The model under review builds one solid part; all positions refer to its coordinate system, in mm. A direction names the side the tool comes from. Round coordinates to 2 decimals unless told otherwise and drop trailing zeros. Order: outer loops, then holes, each group sorted by start corner. A loop starts at its lowest first (then second) coordinate and runs counter-clockwise, first axis right, second up.
1) Mouldability with a two-part tool opening along Z and no side actions: class faces 1 (the face through (30.04, 1.23, 95.38)), 2 (the face through (36, -4, 57.891)), 3 (the face through (-58.047, 1.268, -52.401)) as pulls with the +Z half, pulls with the -Z half, needs draft (parallel to the pull), parting line crosses it, or undercut.
2) Consider section A-A (z = -79). Give the boundary of the cut face in (x, y).
3) To check wall thickness, follow L1, parallel to X at y = 2, z = -38; L2, parallel to Z at x = 14.51, y = 3.95; L3, parallel to Z at x = -30.5, y = 0.5. State the ranges of each line that lie inside material, in increasing order.
4) Consider section B-B (z = 37). Give the number of separate pieces and of enclosed holes in the cut face, then the cut area to 3 significant figures.
5) Clearance check with flat-ended pins moving along their axes: P1, Ø5, axis at x = 13.5, z = -23.5, coming from the -Y side; P2, Ø1.2, axis at x = 37.5, y = 1, coming from the -Z side; P3, Ø1.5, axis at y = 3, z = 26, coming from the -X side. State where each tip first meets the part, or that it passes through.
6) Machinability: for faces 4 (the face through (39, -3, 43)), 5 (the face through (-36.06, 1.27, 35.72)), 6 (the face through (0, 1, -55)), 7 (the face through (14, 5, 6.35)), which of the approach directions +Z, -Z, +X, -X, +Y, -Y give a long, thin tool a straight path to every point of the face, cutting with its end or side? Answer none if there is none.
from build123d import *

# Parameters (mm, degrees)
IZIM1_R                     = 100
IZIM1_W                     = 64
IZIM1_H                     = 64
Y_KSEKLIK_EKSTR_ZYON1_DEPTH = 2.5
KES_EKSTR_ZYON1_DEPTH       = 142.443451598
IZIM3_W                     = 4.7
IZIM3_H                     = 12.7
IZIM3_R                     = 1
Y_KSEKLIK_EKSTR_ZYON2_DEPTH = 5.85
IZIM4_W                     = 4
IZIM4_H                     = 30
Y_KSEKLIK_EKSTR_ZYON3_DEPTH = 4
Y_KSEKLIK_EKSTR_ZYON4_START = 4
IZIM4_3_W                   = 3
IZIM4_3_H                   = 30
IZIM4_3_W_2                 = 4
Y_KSEKLIK_EKSTR_ZYON4_DEPTH = 3
IZIM5_R                     = 3
Y_KSEKLIK_EKSTR_ZYON5_DEPTH = 3
Y_KSEKLIK_EKSTR_ZYON6_START = 3
IZIM5_3_R                   = 5
Y_KSEKLIK_EKSTR_ZYON6_DEPTH = 2
IZIM11_R                    = 1
KES_EKSTR_ZYON5_DEPTH       = 142.667648036
IZIM12_R                    = 5.7
KES_EKSTR_ZYON6_DEPTH       = 142.667648036
KES_EKSTR_ZYON7_DEPTH       = 142.740079018
KES_EKSTR_ZYON8_DEPTH       = 40


with BuildPart() as part:
    # Çizim1 → Yükseklik-Ekstrüzyon1 (new body)
    with BuildSketch(Plane(origin=(0, 0, 0), x_dir=(1, 0, 0), z_dir=(0, 1, 0))):
        with Locations(Location((0, 0, 0), (0, 0, 270))):
            Circle(IZIM1_R)
        with Locations((0, -48)):
            Rectangle(IZIM1_W, IZIM1_H, mode=Mode.SUBTRACT)
    extrude(amount=Y_KSEKLIK_EKSTR_ZYON1_DEPTH)

    # Çizim2 → Kes-Ekstrüzyon1 (cut, through all)
    with BuildSketch(Plane.XZ):
        with BuildLine():
            ThreePointArc((1.17075, 1.767705982), (-11.89, 0), (1.17075, -1.767705982))
            ThreePointArc((1.17075, -1.767705982), (2.785, 0), (1.17075, 1.767705982))
        make_face()
        with BuildLine():
            ThreePointArc((0.78075, 1.254220649), (-11.39, 0), (0.78075, -1.254220649))
            ThreePointArc((0.78075, -1.254220649), (2.285, 0), (0.78075, 1.254220649))
        make_face(mode=Mode.SUBTRACT)
        with BuildLine():
            ThreePointArc((0.78075, -1.254220649), (2.285, 0), (0.78075, 1.254220649))
            ThreePointArc((0.78075, 1.254220649), (-11.39, 0), (0.78075, -1.254220649))
        make_face()
    extrude(amount=-KES_EKSTR_ZYON1_DEPTH, mode=Mode.SUBTRACT)

    # Çizim3 → Yükseklik-Ekstrüzyon2 (add)
    with BuildSketch(Plane(origin=(0, 2.5, 0), x_dir=(1, 0, 0), z_dir=(0, 1, 0))):
        with Locations((-14.24, 0)):
            Rectangle(IZIM3_W, IZIM3_H)
        with Locations((-14.49, 0)):
            Circle(IZIM3_R, mode=Mode.SUBTRACT)
        with Locations((14.26, 0)):
            Rectangle(IZIM3_W, IZIM3_H)
        with Locations((14.51, 0)):
            Circle(IZIM3_R, mode=Mode.SUBTRACT)
    extrude(amount=Y_KSEKLIK_EKSTR_ZYON2_DEPTH)

    # Çizim4 → Yükseklik-Ekstrüzyon3 (add)
    with BuildSketch(Plane.XZ):
        with Locations((37, 42.891487162)):
            Rectangle(IZIM4_W, IZIM4_H)
    extrude(amount=Y_KSEKLIK_EKSTR_ZYON3_DEPTH)

    # Çizim4<3> → Yükseklik-Ekstrüzyon4 (add)
    with BuildSketch(Plane.XZ.offset(Y_KSEKLIK_EKSTR_ZYON4_START)):
        with Locations((33.5, 42.891487162)):
            Rectangle(IZIM4_3_W, IZIM4_3_H)
        with Locations((37, 42.891487162)):
            Rectangle(IZIM4_3_W_2, IZIM4_3_H)
    extrude(amount=Y_KSEKLIK_EKSTR_ZYON4_DEPTH)

    # Çizim5 → Yükseklik-Ekstrüzyon5 (add)
    with BuildSketch(Plane.XZ):
        with Locations(Location((-21.143733637, -10.434588388, 0), (0, 0, 90))):
            Circle(IZIM5_R)
    extrude(amount=Y_KSEKLIK_EKSTR_ZYON5_DEPTH)

    # Çizim5<3> → Yükseklik-Ekstrüzyon6 (add)
    with BuildSketch(Plane.XZ.offset(Y_KSEKLIK_EKSTR_ZYON6_START)):
        with Locations(Location((-21.143733637, -10.434588388, 0), (0, 0, 270))):
            Circle(IZIM5_3_R)
    extrude(amount=Y_KSEKLIK_EKSTR_ZYON6_DEPTH)

    # Çizim11 → Kes-Ekstrüzyon5 (cut, through all)
    with BuildSketch(Plane.XZ):
        with Locations(Location((-59.798043504, -34.469478679, 0), (0, 0, 270))):
            Circle(IZIM11_R)
    extrude(amount=-KES_EKSTR_ZYON5_DEPTH, mode=Mode.SUBTRACT)

    # Çizim12 → Kes-Ekstrüzyon6 (cut, through all)
    with BuildSketch(Plane.XZ):
        with Locations(Location((-64.455689055, 62.812929787, 0), (0, 0, 270))):
            Circle(IZIM12_R)
        with Locations(Location((62.812929787, 64.455689055, 0), (0, 0, 270))):
            Circle(IZIM12_R)
        with Locations(Location((64.455689055, -62.812929787, 0), (0, 0, 270))):
            Circle(IZIM12_R)
        with Locations(Location((-62.812929787, -64.455689055, 0), (0, 0, 270))):
            Circle(IZIM12_R)
    extrude(amount=-KES_EKSTR_ZYON6_DEPTH, mode=Mode.SUBTRACT)

    # Çizim13 → Kes-Ekstrüzyon7 (cut, through all)
    with BuildSketch(Plane(origin=(0, 2.5, 0), x_dir=(1, 0, 0), z_dir=(0, 1, 0))):
        with BuildLine():
            Line((49.903008022, 41.649607326), (42.716090382, 34.645860105))
            ThreePointArc((42.716090382, 34.645860105), (51.838137365, 18.379540649), (55, 0))
            ThreePointArc((55, 0), (52.962250707, -14.832396974), (47, -28.565713714))
            Line((47, -28.565713714), (47, -41.065070429))
            Line((47, -41.065070429), (48.811350554, -42.923793601))
            ThreePointArc((48.811350554, -42.923793601), (60.81832695, -22.937547973), (65, 0))
            ThreePointArc((65, 0), (61.109309935, 22.150671306), (49.903008022, 41.649607326))
        make_face()
        with BuildLine():
            Line((35.517896602, 27.631124135), (28.298613495, 20.595836333))
            ThreePointArc((28.298613495, 20.595836333), (29.153169835, 19.367309792), (29.954428374, 18.10337595))
            Line((29.954428374, 18.10337595), (40, 18.10337595))
            Line((40, 18.10337595), (40, -19.891487162))
            Line((40, -19.891487162), (40.364944426, -19.891487162))
            ThreePointArc((40.364944426, -19.891487162), (43.825919837, -10.212186368), (45, 0))
            ThreePointArc((45, 0), (42.563513407, 14.606413881), (35.517896602, 27.631124135))
        make_face()
        with BuildLine():
            Line((61.743044694, 53.187881186), (57.083186115, 48.646786769))
            ThreePointArc((57.083186115, 48.646786769), (70.37840208, 25.920658184), (75, 0))
            ThreePointArc((75, 0), (70.037988798, -26.826854551), (55.808529997, -50.103971694))
            Line((55.808529997, -50.103971694), (60.349624415, -54.763830273))
            ThreePointArc((60.349624415, -54.763830273), (62.697904283, -54.45635062), (65.052635888, -54.709730067))
            ThreePointArc((65.052635888, -54.709730067), (79.85760468, -29.116369533), (85, 0))
            ThreePointArc((85, 0), (80.226750198, 28.083243272), (66.443092878, 53.012408064))
            ThreePointArc((66.443092878, 53.012408064), (64.082605735, 52.819891769), (61.743044694, 53.187881186))
        make_face()
        with BuildLine():
            Line((-53.187881186, 61.743044694), (-48.646786769, 57.083186115))
            ThreePointArc((-48.646786769, 57.083186115), (0.968005182, 74.993752846), (50.103971694, 55.808529997))
            Line((50.103971694, 55.808529997), (54.763830273, 60.349624415))
            ThreePointArc((54.763830273, 60.349624415), (54.45635062, 62.697904283), (54.709730067, 65.052635888))
            ThreePointArc((54.709730067, 65.052635888), (1.097072539, 84.992919892), (-53.012408064, 66.443092878))
            ThreePointArc((-53.012408064, 66.443092878), (-52.862924329, 65.454383896), (-52.812929787, 64.455689055))
            ThreePointArc((-52.812929787, 64.455689055), (-52.907111143, 63.086471397), (-53.187881186, 61.743044694))
        make_face()
        with BuildLine():
            Line((-41.649607326, 49.903008022), (-34.645860105, 42.716090382))
            ThreePointArc((-34.645860105, 42.716090382), (0.709870466, 54.995418754), (35.736875962, 41.807603334))
            Line((35.736875962, 41.807603334), (42.923793601, 48.811350554))
            ThreePointArc((42.923793601, 48.811350554), (0.838937824, 64.9945858), (-41.649607326, 49.903008022))
        make_face()
        with BuildLine():
            Line((-27.631124135, 35.517896602), (-20.595836333, 28.298613495))
            ThreePointArc((-20.595836333, 28.298613495), (0.451735751, 34.997084662), (21.319399074, 27.757579562))
            Line((21.319399074, 27.757579562), (28.538682181, 34.792867363))
            ThreePointArc((28.538682181, 34.792867363), (0.580803109, 44.996251708), (-27.631124135, 35.517896602))
        make_face()
        with BuildLine():
            Line((-13.514642522, 21.032223789), (-10.660441189, 18.10337595))
            Line((-10.660441189, 18.10337595), (11.412707121, 18.10337595))
            Line((11.412707121, 18.10337595), (14.053009368, 20.676385751))
            ThreePointArc((14.053009368, 20.676385751), (0.322668394, 24.997917615), (-13.514642522, 21.032223789))
        make_face()
        with BuildLine():
            Line((-40, 18.10337595), (-29.954428374, 18.10337595))
            ThreePointArc((-29.954428374, 18.10337595), (-28.900772761, 19.741968844), (-27.757579562, 21.319399074))
            Line((-27.757579562, 21.319399074), (-34.792867363, 28.538682181))
            ThreePointArc((-34.792867363, 28.538682181), (-44.74960726, 4.740532682), (-40, -20.615528128))
            Line((-40, -20.615528128), (-40, 18.10337595))
        make_face()
        with BuildLine():
            Line((-49.903008022, -41.649607326), (-42.716090382, -34.645860105))
            ThreePointArc((-42.716090382, -34.645860105), (-54.995418754, 0.709870466), (-41.807603334, 35.736875962))
            Line((-41.807603334, 35.736875962), (-48.811350554, 42.923793601))
            ThreePointArc((-48.811350554, 42.923793601), (-64.9945858, 0.838937824), (-49.903008022, -41.649607326))
        make_face()
        with BuildLine():
            Line((-61.743044694, -53.187881186), (-57.083186115, -48.646786769))
            ThreePointArc((-57.083186115, -48.646786769), (-74.993752846, 0.968005182), (-55.808529997, 50.103971694))
            Line((-55.808529997, 50.103971694), (-60.349624415, 54.763830273))
            ThreePointArc((-60.349624415, 54.763830273), (-62.697904283, 54.45635062), (-65.052635888, 54.709730067))
            ThreePointArc((-65.052635888, 54.709730067), (-84.992919892, 1.097072539), (-66.443092878, -53.012408064))
            ThreePointArc((-66.443092878, -53.012408064), (-64.082605735, -52.819891769), (-61.743044694, -53.187881186))
        make_face()
        with BuildLine():
            Line((-40, -75), (-40, -63.442887702))
            ThreePointArc((-40, -63.442887702), (-45.213408223, -59.839349235), (-50.103971694, -55.808529997))
            Line((-50.103971694, -55.808529997), (-54.763830273, -60.349624415))
            ThreePointArc((-54.763830273, -60.349624415), (-54.533023389, -61.571677963), (-54.455689055, -62.812929787))
            ThreePointArc((-54.455689055, -62.812929787), (-54.519402277, -63.939963533), (-54.709730067, -65.052635888))
            ThreePointArc((-54.709730067, -65.052635888), (-47.615341599, -70.411499376), (-40, -75))
        make_face()
        with BuildLine():
            Line((-40, -51.23475383), (-40, -45.962074643))
            Line((-40, -45.962074643), (-42.923793601, -48.811350554))
            ThreePointArc((-42.923793601, -48.811350554), (-41.479598686, -50.044409207), (-40, -51.23475383))
        make_face()
        with BuildLine():
            ThreePointArc((48.646786769, -57.083186115), (47.828251585, -57.770739569), (47, -58.446556785))
            Line((47, -58.446556785), (47, -65.891487162))
            Line((47, -65.891487162), (40, -65.891487162))
            Line((40, -65.891487162), (40, -75))
            ThreePointArc((40, -75), (46.702592844, -71.020193056), (53.012408064, -66.443092878))
            ThreePointArc((53.012408064, -66.443092878), (52.819891769, -64.082605735), (53.187881186, -61.743044694))
            Line((53.187881186, -61.743044694), (48.646786769, -57.083186115))
        make_face()
    extrude(amount=-KES_EKSTR_ZYON7_DEPTH, mode=Mode.SUBTRACT)

    # Çizim14 → Kes-Ekstrüzyon8 (cut)
    with BuildSketch(Plane.XY.offset(16)):
        Polygon((-32, 0), (-32, 2.5), (-40, 2.5), align=None)
        Polygon((32, 2.5), (32, 0), (40, 2.5), align=None)
    extrude(amount=KES_EKSTR_ZYON8_DEPTH, mode=Mode.SUBTRACT)


solid = part.part
Answer below:
1. face 1: parting line crosses it
1. face 2: pulls with the +Z half
1. face 3: undercut
2. outline: (-61.31, 0) - (-31.37, 0) - (-31.37, 2.5) - (-61.31, 2.5) - close; (31.37, 0) - (61.31, 0) - (61.31, 2.5) - (31.37, 2.5) - close
3. L1: x = -92.5 to -76.03, -64.66 to -52.74, -44.01 to -24.1, 24.1 to 46.16, 52.74 to 64.66, 76.03 to 92.5
3. L2: z = -6.35 to -1, 1 to 6.35
3. L3: z = -95.24 to -79.34, -68.52 to -57.4, -45.77 to -24.13, -18.1 to 16, 80 to 95.24
4. separate pieces: 6
4. enclosed holes: 0
4. area: 228 mm2
5. P1: stops at y = 0
5. P2: stops at z = -92.94
5. P3: stops at x = -96.71
6. face 4: +Z, -Z, +X, -Y
6. face 5: +Y
6. face 6: +Y, -Y
6. face 7: +Z, +X, -X, +Y
